Geometry: see drawing. Coordinates: mm, zero at the bounding-box minimum. A direction names the side the tool comes from. Coordinates: 2 decimals unless noted, no trailing zeros. Loops run counter-clockwise (first coordinate to the right, second up) from the corner with the lowest first, then second, coordinate; pieces in that order, holes last. Notation, with made-up numbers: (-9.75, -37.75) -> (32.25, -37.75) arc R7 ccw to (32.25, -33.75) -> close; hole circle Ø1 at (-20, -9.75). An arc over 180 degrees is marked (long way). Answer as a JSON object with one key per item and string values.
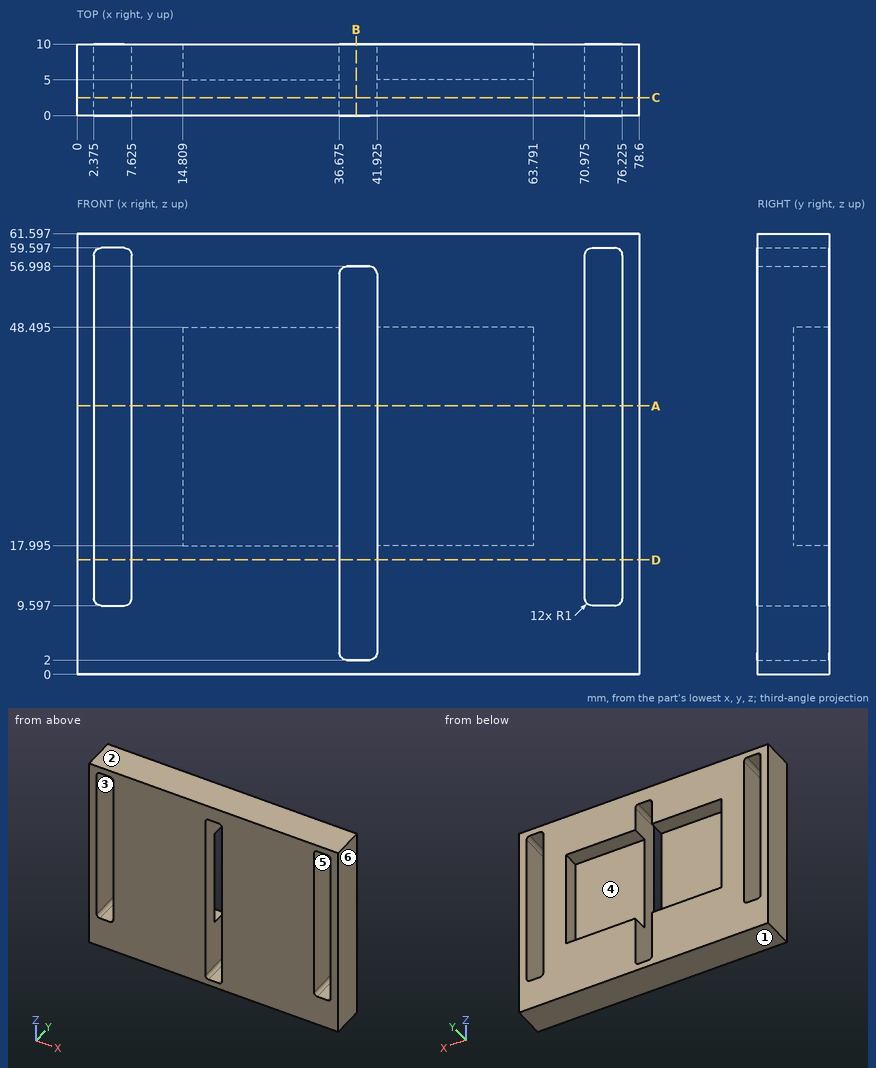
1. Mould query, pull axis Z, two halves, no side actions, for the marked faces 1, 2 and 3. Classes: pulls with the +Z half, pulls with the -Z half, needs draft (parallel to the pull), parting line crosses it, or undercut.
Reply:
{"face 1": "pulls with the -Z half", "face 2": "pulls with the +Z half", "face 3": "undercut"}
2. Access query for the marked faces 4, 5 and 6. Directions: +Z, -Z, +X, -X, +Y, -Y. A direction counts if a zero-diameter tool reaches every point of the face in a straight line with its end or side. Return the directions, or none.
Reply:
{"face 4": "+Y", "face 5": "+Y, -Y", "face 6": "+Z, -Z, +X, +Y, -Y"}
3. Line query: line 1 along X through (y, z) = (5.5, 19) (1 decimal); line 2 along X through (y, z) = (3.5, 21.5) (1 decimal); line 3 along X through (y, z) = (7.5, 4.5) (1 decimal). Output: solid intervals per line, ascending.
Reply:
{"line 1": "x = 0 to 2.4, 7.6 to 14.8, 63.8 to 71, 76.2 to 78.6", "line 2": "x = 0 to 2.4, 7.6 to 36.7, 41.9 to 71, 76.2 to 78.6", "line 3": "x = 0 to 36.7, 41.9 to 78.6"}
4. Section query D-D (z = 16). Return loops of the section in (x, y) (1 decimal).
Reply:
{"outline": "(0, 0) -> (2.4, 0) -> (2.4, 10) -> (0, 10) -> close; (7.6, 0) -> (36.7, 0) -> (36.7, 10) -> (7.6, 10) -> close; (41.9, 0) -> (71, 0) -> (71, 10) -> (41.9, 10) -> close; (76.2, 0) -> (78.6, 0) -> (78.6, 10) -> (76.2, 10) -> close"}
5. Section query B-B (x = 39). Return loops of the section in (y, z).
Reply:
{"outline": "(0, 0) -> (10, 0) -> (10, 2) -> (0, 2) -> close; (0, 57) -> (10, 57) -> (10, 61.6) -> (0, 61.6) -> close"}
6. Section query C-C (y = 2.5). Return loops of the section in (x, z) (1 decimal), plus the area to 3 significant figures.
Reply:
{"outline": "(0, 0) -> (78.6, 0) -> (78.6, 61.6) -> (0, 61.6) -> close; hole (2.4, 10.6) arc R1 ccw to (3.4, 9.6) -> (6.6, 9.6) arc R1 ccw to (7.6, 10.6) -> (7.6, 58.6) arc R1 ccw to (6.6, 59.6) -> (3.4, 59.6) arc R1 ccw to (2.4, 58.6) -> close; hole (36.7, 3) arc R1 ccw to (37.7, 2) -> (40.9, 2) arc R1 ccw to (41.9, 3) -> (41.9, 56) arc R1 ccw to (40.9, 57) -> (37.7, 57) arc R1 ccw to (36.7, 56) -> close; hole (71, 10.6) arc R1 ccw to (72, 9.6) -> (75.2, 9.6) arc R1 ccw to (76.2, 10.6) -> (76.2, 58.6) arc R1 ccw to (75.2, 59.6) -> (72, 59.6) arc R1 ccw to (71, 58.6) -> close", "area": "4,030 mm2"}
7. Section query A-A (z = 37.5). Return loops of the section in (x, y) (1 decimal).
Reply:
{"outline": "(0, 0) -> (2.4, 0) -> (2.4, 10) -> (0, 10) -> close; (7.6, 0) -> (36.7, 0) -> (36.7, 5) -> (14.8, 5) -> (14.8, 10) -> (7.6, 10) -> close; (41.9, 0) -> (71, 0) -> (71, 10) -> (63.8, 10) -> (63.8, 5) -> (41.9, 5) -> close; (76.2, 0) -> (78.6, 0) -> (78.6, 10) -> (76.2, 10) -> close"}
8. Pin query (flat end, axial travel): P1, Ø1.5, axis at y = 6.5, z = 34.5, coming from the -X side; P2, Ø6.5, axis at x = 27.5, z = 34, coming from the +Y side. Return the tip coordinate at first contact, or that it passes through.
Reply:
{"P1": "stops at x = 0", "P2": "stops at y = 5"}
